Model file for the job. Use its own axes, mm. A direction names the side the tool comes from. Round coordinates to 2 decimals unless told otherwise and drop trailing zeros. Loops run counter-clockwise (first coordinate to the right, second up) from the corner with the lowest first, then second, coordinate; pieces in that order, holes last. Notation, with made-up numbers: (-17, -1.5) -> (26, -1.5) arc R17 cw to (26, 8.5) -> close; hole circle Ø2 at (-39.75, 85). An arc over 180 degrees is marked (long way). Use a Markdown table: item, result.
from build123d import *

# Parameters (mm, degrees)
F1_DEPTH = 25.4
F2_DEPTH = 3.175
F3_R     = 5.08
F5_DEPTH = 25.4


# Not quite as in the source:
# - a feature names something its author has since deleted; it is built from what else it names


with BuildPart() as f1:
    # F0 (on Top) → F1 (new body)
    with BuildSketch(Plane.XY):
        Polygon((-77.7875, -1.5875), (77.7875, -1.5875), (77.7875, 1.5875), (0, 1.5875), (-77.7875, 1.5875), align=None)
    extrude(amount=F1_DEPTH)

    # F0 (on Top) → F2 (join)
    with BuildSketch(Plane.XY):
        Polygon((0, 1.5875), (77.7875, 1.5875), (57.15, 109.5375), (0, 109.5375), (-57.15, 109.5375), (-77.7875, 1.5875), align=None)
        with BuildLine():
            ThreePointArc((14.2875, 39.6875), (10.1027881362, 29.5847118638), (0, 25.4))
            ThreePointArc((0, 25.4), (-10.1027881362, 49.7902881362), (14.2875, 39.6875))
        make_face(mode=Mode.SUBTRACT)
    extrude(amount=F2_DEPTH)

    # F3
    f3_edges = [f1.edges().sort_by_distance(p)[0] for p in [
        (-77.7875, 0, 25.4),
        (77.7875, 0, 25.4),
        (0, -1.5875, 0),
        (57.15, 109.5375, 1.5875),
        (-57.15, 109.5375, 1.5875),
    ]]
    fillet(f3_edges, radius=F3_R)

    # F4 (on face) → F5 (cut)
    with BuildSketch(Plane.XZ.offset(1.5875)):
        with BuildLine():
            ThreePointArc((-71.4375, 19.05), (-73.6825640303, 18.1200640303), (-74.6125, 15.875))
            ThreePointArc((-74.6125, 15.875), (-73.6825640303, 13.6299359697), (-71.4375, 12.7))
            Line((-71.4375, 12.7), (-61.9125, 12.7))
            ThreePointArc((-61.9125, 12.7), (-59.6674359697, 13.6299359697), (-58.7375, 15.875))
            ThreePointArc((-58.7375, 15.875), (-59.6674359697, 18.1200640303), (-61.9125, 19.05))
            Line((-61.9125, 19.05), (-71.4375, 19.05))
        make_face()
        with BuildLine():
            ThreePointArc((46.0375, 15.875), (45.1075640303, 18.1200640303), (42.8625, 19.05))
            Line((42.8625, 19.05), (33.3375, 19.05))
            ThreePointArc((33.3375, 19.05), (31.0924359697, 18.1200640303), (30.1625, 15.875))
            ThreePointArc((30.1625, 15.875), (31.0924359697, 13.6299359697), (33.3375, 12.7))
            Line((33.3375, 12.7), (42.8625, 12.7))
            ThreePointArc((42.8625, 12.7), (45.1075640303, 13.6299359697), (46.0375, 15.875))
        make_face()
    extrude(amount=-F5_DEPTH, mode=Mode.SUBTRACT)


solid = f1.part
Q1. Band-saw the part on B-B, the plane y = 48.5. Give the cut face in (x, z) (3 decimals).
Results list:
| item | result |
|---|---|
| outline | (-68.819, 0) -> (-11.246, 0) -> (-11.246, 3.175) -> (-68.819, 3.175) -> close; (11.246, 0) -> (68.819, 0) -> (68.819, 3.175) -> (11.246, 3.175) -> close |
Q2. Band-saw the part on C-C, the plane x = 21. Give the cut face in (y, z) (1 decimal).
Results list:
| item | result |
|---|---|
| outline | (-1.6, 5.1) arc R5.1 ccw to (3.5, 0) -> (109.5, 0) -> (109.5, 3.2) -> (1.6, 3.2) -> (1.6, 25.4) -> (-1.6, 25.4) -> close |
Q3. Tool access for faces 4 (the face through (76.34, 0.02, 23.87)), 5 (the face through (1, 1.588, 14)), 6 (the face through (-67, 0, 19.05)): list every direction of +Z, -Z, +X, -X, +Y, -Y with a clear straight run to the whole face (end or side of a thin tool).
Results list:
| item | result |
|---|---|
| face 4 | +Z, +X, +Y, -Y |
| face 5 | +Z, +X, -X, +Y |
| face 6 | +Y, -Y |
Q4. Band-saw the part on D-D, the plane y = 15. Give the cut face in (x, z) (3 decimals), plus the area to 3 significant figures.
Results list:
| item | result |
|---|---|
| outline | (-75.223, 0) -> (75.223, 0) -> (75.223, 3.175) -> (-75.223, 3.175) -> close |
| area | 478 mm² |
Q5. Pull direction Z, two halves, no side cores. Call faces 1 (the face through (-1, 56, 3.175)), 2 (the face through (-77.788, 0, 10)), 3 (the face through (-67, 0, 12.7)): released by +Z, released by -Z, zero draft, split by the parting line, or undercut.
Results list:
| item | result |
|---|---|
| face 1 | released by +Z |
| face 2 | zero draft |
| face 3 | undercut |
Q6. Drill centre lines: L1, parallel to Z at x = -28, y = 6 (3 decimals); L2, parallel to Y at x = -55.5, z = 11.75. Where is each one in solid material? Low to high. Write a range as from..to.
Results list:
| item | result |
|---|---|
| L1 | z = 0..3.175 |
| L2 | y = -1.59..1.59 |
Q7. Flat gauge pins, fed straight in: pin 1 (1 mm diameter, centred on x = -66.5, y = 0, fed in from -Z); pin 2 (5 mm diameter, centred on x = 34.5, z = 7, fed in from +Y); pin 3 (1 mm diameter, centred on x = 38, y = -0.5, fed in from -Z). Where does each tip first touch, or does it go through?
Results list:
| item | result |
|---|---|
| pin 1 | stops at z = 0.97 |
| pin 2 | stops at y = 1.59 |
| pin 3 | stops at z = 1.39 |
Q8. Band-saw the part on A-A, the plane x = 0. Give the cut face in (y, z) (1 decimal), plus the area to 3 significant figures.
Results list:
| item | result |
|---|---|
| outline | (-1.6, 5.1) arc R5.1 ccw to (3.5, 0) -> (25.4, 0) -> (25.4, 3.2) -> (1.6, 3.2) -> (1.6, 25.4) -> (-1.6, 25.4) -> close; (54, 0) -> (109.5, 0) -> (109.5, 3.2) -> (54, 3.2) -> close |
| area | 327 mm² |
